Could you check a few things on this model? Use its own coordinates, in mm. A direction names the side the tool comes from. Coordinates: 2 decimals unless noted, no trailing zeros. Loops run counter-clockwise (first coordinate to the right, second up) from the corner with the lowest first, then second, coordinate; pieces in that order, holes last.
from build123d import *

# Parameters (mm, degrees)
F1_DEPTH     = 4
F3_DEPTH     = 25
F4_R         = 2
F5_W         = 5.058165174
F5_H         = 1.9329627007
F6_DEPTH     = 1
F7_R         = 1.5
F8_W         = 5.058165174
F8_H         = 1.4937128872
F9_DEPTH     = 1
F10_T1_DEPTH = 12.1292329858


# Not quite as in the source:
# - a fillet or chamfer that OpenCascade refuses, or shapes differently, is made with other operations: its cross-section is extruded or revolved along the edge and cut away or added


with BuildPart() as f1:
    # F0 (on Top) → F1 (new body)
    with BuildSketch(Plane.XY):
        with BuildLine():
            ThreePointArc((2.7663980634, -1.7057378916), (3.1267629992, -0.8864835853), (3.25, 0))
            ThreePointArc((3.25, 0), (3.1267629992, 0.8864835853), (2.7663980634, 1.7057378916))
            ThreePointArc((2.7663980634, 1.7057378916), (2.2980970389, 2.2980970389), (1.7057378916, 2.7663980634))
            ThreePointArc((1.7057378916, 2.7663980634), (0, 3.25), (-1.7057378916, 2.7663980634))
            ThreePointArc((-1.7057378916, 2.7663980634), (-2.2980970389, 2.2980970389), (-2.7663980634, 1.7057378916))
            ThreePointArc((-2.7663980634, 1.7057378916), (-3.25, 0), (-2.7663980634, -1.7057378916))
            ThreePointArc((-2.7663980634, -1.7057378916), (-2.2980970389, -2.2980970389), (-1.7057378916, -2.7663980634))
            ThreePointArc((-1.7057378916, -2.7663980634), (0, -3.25), (1.7057378916, -2.7663980634))
            ThreePointArc((1.7057378916, -2.7663980634), (2.2980970389, -2.2980970389), (2.7663980634, -1.7057378916))
        make_face()
        with BuildLine():
            ThreePointArc((1.7057378916, 2.7663980634), (2.2980970389, 2.2980970389), (2.7663980634, 1.7057378916))
            Line((2.7663980634, 1.7057378916), (4.2426406871, 3.1819805153))
            Line((4.2426406871, 3.1819805153), (3.7123106012, 3.7123106012))
            Line((3.7123106012, 3.7123106012), (3.1819805153, 4.2426406871))
            Line((3.1819805153, 4.2426406871), (1.7057378916, 2.7663980634))
        make_face()
        with BuildLine():
            Line((4.2426406871, -3.1819805153), (2.7663980634, -1.7057378916))
            ThreePointArc((2.7663980634, -1.7057378916), (2.2980970389, -2.2980970389), (1.7057378916, -2.7663980634))
            Line((1.7057378916, -2.7663980634), (3.1819805153, -4.2426406871))
            Line((3.1819805153, -4.2426406871), (3.7123106012, -3.7123106012))
            Line((3.7123106012, -3.7123106012), (4.2426406871, -3.1819805153))
        make_face()
        with BuildLine():
            ThreePointArc((-2.7663980634, 1.7057378916), (-2.2980970389, 2.2980970389), (-1.7057378916, 2.7663980634))
            Line((-1.7057378916, 2.7663980634), (-3.1819805153, 4.2426406871))
            Line((-3.1819805153, 4.2426406871), (-3.7123106012, 3.7123106012))
            Line((-3.7123106012, 3.7123106012), (-4.2426406871, 3.1819805153))
            Line((-4.2426406871, 3.1819805153), (-2.7663980634, 1.7057378916))
        make_face()
        with BuildLine():
            Line((-3.1819805153, -4.2426406871), (-1.7057378916, -2.7663980634))
            ThreePointArc((-1.7057378916, -2.7663980634), (-2.2980970389, -2.2980970389), (-2.7663980634, -1.7057378916))
            Line((-2.7663980634, -1.7057378916), (-4.2426406871, -3.1819805153))
            Line((-4.2426406871, -3.1819805153), (-3.7123106012, -3.7123106012))
            Line((-3.7123106012, -3.7123106012), (-3.1819805153, -4.2426406871))
        make_face()
    extrude(amount=F1_DEPTH)

    # F2 (on face) → F3 (join)
    with BuildSketch(Plane.XY.offset(4)):
        Polygon((-1.5528574586, 2.6730068494), (-2.529082587, 0.9646130493), (2.529082587, 0.9646130493), (1.5528574586, 2.6730068494), (0, 3.0187531374), align=None)
        Polygon((2.529082587, -0.9646130493), (-2.529082587, -0.9646130493), (-1.5528574586, -2.6730068494), (0, -3.0187531374), (1.5528574586, -2.6730068494), align=None)
    extrude(amount=F3_DEPTH)

    # F4
    f4_edges = [f1.edges().sort_by_distance(p)[0] for p in [
        (0, -0.964613, 29),
    ]]
    fillet(f4_edges, radius=F4_R)

    # F5 (on face) → F6 (join)
    with BuildSketch(Plane.XZ.offset(-0.9646130493)):
        with Locations((0, 28.0335186496)):
            Rectangle(F5_W, F5_H)
    extrude(amount=F6_DEPTH)

    # F7
    f7_edges = [f1.edges().sort_by_distance(p)[0] for p in [
        (0, -0.035387, 29),
    ]]
    fillet(f7_edges, radius=F7_R)

    # F8 (on face) → F9 (join)
    with BuildSketch(Plane.XZ.offset(-0.9646130493)):
        with Locations((0, 18.9132643864)):
            Rectangle(F8_W, F8_H)
    extrude(amount=F9_DEPTH)

    # F10: fillet of radius 1.5 on 1 edges, made by hand

    # F10_s2 → F10_t1 (cut)
    with BuildSketch(Plane.YZ.offset(-6.0646164929)):
        with BuildLine():
            ThreePointArc((0.9646130493, 19.6601208299), (0.2398681779, 19.1119326714), (-0.0353869507, 18.2459072676))
            Line((-0.0353869507, 18.2459072676), (-0.0353869507, 19.6601208299))
            Line((-0.0353869507, 19.6601208299), (0.9646130493, 19.6601208299))
        make_face()
    extrude(amount=F10_T1_DEPTH, mode=Mode.SUBTRACT)


solid = f1.part
1) Imagine slicing it at A-A on z = 7.5. List the corners of the cut face in (x, y) for me.
2) Will these pins go through, and if not, where does the flat tip stop? pin 1 (4 mm diameter, centred on y = 1.5, z = 9, fed in from -X); pin 2 (2.5 mm diameter, centred on x = -1, z = 21.5, fed in from -Y); pin 3 (2 mm diameter, centred on y = 2.5, z = 10, fed in from +X).
3) Imagine slicing it at C-C on x = -1. List the corners of the cut face in (y, z) for me, plus the area to 3 significant figures.
4) Imagine slicing it at B-B on z = 3. List the corners of the cut face in (x, y) for me, plus the area to 3 significant figures.
5) If I drill on L1, parallel to Z at x = -3.5, y = 3; L2, parallel to Z at x = -1.5, y = 0.75; L3, parallel to Y at x = 2.25, z = 27, over which ranges is the centre line in solid material (lowest first)?
6) We'd pull the mould along Z, two halves only. Please class faces 5 (the flat face through (0, 0.965, 23)), 6 (the flat face through (2.048, 1.807, 16.325)), 7 (the cylindrical face through (0.035, 0.416, 28.572)): released by +Z, released by -Z, zero draft, split by the parting line, or undercut.
7) For faces 1 (the flat face through (-2.034, 1.831, 16.325)), 2 (the cylindrical face through (-0.035, -1.314, 28.129)), 3 (the flat face through (-2.048, -1.807, 16.314)), 4 (the flat face through (0, 0.965, 11)), which set-ups out of +Z, -Z, +X, -X, +Y, -Y let a thin tool reach every point of the face, with its end or its side?
8) Imagine slicing it at D-D on z = 18.75. List the corners of the cut face in (x, y) for me.
Solved:
1. outline: (-2.53, -0.96) - (-1.55, -2.67) - (0, -3.02) - (1.55, -2.67) - (2.53, -0.96) - close; (-2.53, 0.96) - (2.53, 0.96) - (1.55, 2.67) - (0, 3.02) - (-1.55, 2.67) - close
2. pin 1: stops at x = -2.53
2. pin 2: stops at y = -3.02
2. pin 3: stops at x = 2.22
3. outline: (-3.09, 0) - (3.09, 0) - (3.09, 4) - (2.8, 4) - (2.8, 29) - (1.46, 29) arc R1.5 ccw to (-0.04, 27.5) - (-0.04, 27.07) - (0.96, 27.07) - (0.96, 19.66) arc R1.5 ccw to (-0.04, 18.25) - (-0.04, 18.17) - (0.96, 18.17) - (0.96, 4) - (-0.96, 4) - (-0.96, 27) arc R2 ccw to (-2.8, 28.99) - (-2.8, 4) - (-3.09, 4) - close
3. area: 118 mm2
4. outline: (-4.24, -3.18) - (-3.18, -4.24) - (-1.71, -2.77) arc R3.25 ccw to (1.71, -2.77) - (3.18, -4.24) - (4.24, -3.18) - (2.77, -1.71) arc R3.25 ccw to (2.77, 1.71) - (4.24, 3.18) - (3.18, 4.24) - (1.71, 2.77) arc R3.25 ccw to (-1.71, 2.77) - (-3.18, 4.24) - (-4.24, 3.18) - (-2.77, 1.71) arc R3.25 ccw to (-2.77, -1.71) - close
4. area: 45.4 mm2
5. L1: z = 0 to 4
5. L2: z = 0 to 4, 18.17 to 19.56, 27.07 to 28.82
5. L3: y = -1.45 to -0.96, 0.96 to 1.45
6. face 5: undercut
6. face 6: zero draft
6. face 7: released by +Z
7. face 1: +Z, -X, +Y
7. face 2: +Z, +X, -X
7. face 3: +Z, -X, -Y
7. face 4: +X, -X
8. outline: (-2.53, -0.96) - (-1.55, -2.67) - (0, -3.02) - (1.55, -2.67) - (2.53, -0.96) - close; (-2.53, 0.05) - (2.53, 0.05) - (2.53, 0.96) - (1.55, 2.67) - (0, 3.02) - (-1.55, 2.67) - (-2.53, 0.96) - close
